CAD build for the part. Positions are in the model's coordinates, mm. A direction names the side the tool comes from. Give positions to 0.01 mm unless a question says otherwise; leave off trailing zeros. Write each loop counter-clockwise with the first axis right and the second up, starting at its lowest first coordinate (ties: lowest second). Pieces come first, ordered by that corner, then holes. Notation, with made-up numbers: (15.25, 48.5) - (24.25, 48.5) arc R12 ccw to (24.25, 68.5) - close; hole circle Ø5 at (61.5, 63.25). An arc over 180 degrees is marked (long way). Answer as a JSON object with one key per item and string values.
from build123d import *

# Parameters (mm, degrees)
SKETCH1_W            = 115
SKETCH1_H            = 100
BOSS_EXTRUDE1_DEPTH  = 20
SKETCH8_R            = 7
SKETCH8_R_2          = 6
BOSS_EXTRUDE4_DEPTH  = 20
SKETCH9_W            = 200
SKETCH9_H            = 100
BOSS_EXTRUDE5_DEPTH  = 16.6
SKETCH10_R           = 9
SKETCH10_R_2         = 10
BOSS_EXTRUDE7_DEPTH  = 20
SKETCH11_W           = 69.56
SKETCH11_H           = 59.638518518
SKETCH11_W_2         = 62.561838236
SKETCH11_H_2         = 53.638518518
BOSS_EXTRUDE9_DEPTH  = 15
SKETCH17_W           = 20
SKETCH17_H           = 100
BOSS_EXTRUDE15_DEPTH = 20
SKETCH15_R           = 14.1
CUT_EXTRUDE2_DEPTH   = 10
SKETCH21_R           = 1.76744544
SKETCH21_R_2         = 2.038433248
CUT_EXTRUDE3_DEPTH   = 20
SKETCH19_R           = 1.6
CUT_EXTRUDE4_DEPTH   = 38
CUT_EXTRUDE5_DEPTH   = 3
SKETCH23_W           = 7.97749669
SKETCH23_H           = 22.361861783
CUT_EXTRUDE6_DEPTH   = 10
CUT_EXTRUDE7_DEPTH   = 3
CUT_EXTRUDE8_DEPTH   = 3


with BuildPart() as part:
    # Sketch1 → Boss-Extrude1 (new body)
    with BuildSketch(Plane(origin=(0, 0, 0), x_dir=(1, 0, 0), z_dir=(0, 1, 0))):
        Rectangle(SKETCH1_W, SKETCH1_H)
    extrude(amount=BOSS_EXTRUDE1_DEPTH)

    # Sketch8 → Boss-Extrude4 (add)
    with BuildSketch(Plane.XZ):
        with Locations(Location((0, 0, 0), (0, 0, 90))):
            Circle(SKETCH8_R)
        with Locations(Location((42.407889557, -36.876425702, 0), (0, 0, 90))):
            Circle(SKETCH8_R_2)
        with Locations(Location((42.407889557, 36.876425702, 0), (0, 0, 90))):
            Circle(SKETCH8_R_2)
    extrude(amount=BOSS_EXTRUDE4_DEPTH)

    # Sketch9 → Boss-Extrude5 (add)
    with BuildSketch(Plane.XZ.offset(20)):
        with Locations((-42.5, 0)):
            Rectangle(SKETCH9_W, SKETCH9_H)
    extrude(amount=BOSS_EXTRUDE5_DEPTH)

    # Sketch10 → Boss-Extrude7 (add)
    with BuildSketch(Plane.XZ.offset(36.6)):
        with Locations(Location((37.5, -25, 0), (0, 0, 270))):
            Circle(SKETCH10_R)
        with Locations(Location((-122.5, -25, 0), (0, 0, 90))):
            Circle(SKETCH10_R)
        with Locations(Location((-122.5, 25, 0), (0, 0, 270))):
            Circle(SKETCH10_R)
        with Locations(Location((37.5, 25, 0), (0, 0, 90))):
            Circle(SKETCH10_R)
        with Locations(Location((-42.5, 0, 0), (0, 0, 270))):
            Circle(SKETCH10_R_2)
    extrude(amount=BOSS_EXTRUDE7_DEPTH)

    # Sketch11 → Boss-Extrude9 (add)
    with BuildSketch(Plane(origin=(0, 20, 0), x_dir=(1, 0, 0), z_dir=(0, 1, 0))):
        Rectangle(SKETCH11_W, SKETCH11_H)
        Rectangle(SKETCH11_W_2, SKETCH11_H_2, mode=Mode.SUBTRACT)
    extrude(amount=BOSS_EXTRUDE9_DEPTH)

    # Sketch17 → Boss-Extrude15 (add)
    with BuildSketch(Plane.XZ):
        with Locations((-47.5, 0)):
            Rectangle(SKETCH17_W, SKETCH17_H)
    extrude(amount=BOSS_EXTRUDE15_DEPTH)

    # Sketch15 → Cut-Extrude2 (cut)
    with BuildSketch(Plane(origin=(0, -20, 0), x_dir=(1, 0, 0), z_dir=(0, 1, 0))):
        with Locations(Location((-78.6, 0, 0), (0, 0, 270))):
            Circle(SKETCH15_R)
    extrude(amount=-CUT_EXTRUDE2_DEPTH, mode=Mode.SUBTRACT)

    # Sketch21 → Cut-Extrude3 (cut)
    with BuildSketch(Plane(origin=(0, -30, 0), x_dir=(1, 0, 0), z_dir=(0, 1, 0))):
        with Locations(Location((-85.16065049, 0, 0), (0, 0, 270))):
            Circle(SKETCH21_R)
        with Locations(Location((-73.222056531, 0, 0), (0, 0, 270))):
            Circle(SKETCH21_R_2)
    extrude(amount=-CUT_EXTRUDE3_DEPTH, mode=Mode.SUBTRACT)

    # Sketch19 → Cut-Extrude4 (cut)
    with BuildSketch(Plane.ZY.offset(57.5)):
        with Locations((-32.14, -13.409140004)):
            Circle(SKETCH19_R)
        with Locations((32.14, -13.409140004)):
            Circle(SKETCH19_R)
        with Locations((-32.14, 14.690859996)):
            Circle(SKETCH19_R)
        with Locations(Location((32.14, 14.690859996, 0), (0, 0, 180))):
            Circle(SKETCH19_R)
    extrude(amount=-CUT_EXTRUDE4_DEPTH, mode=Mode.SUBTRACT)

    # Sketch22 → Cut-Extrude5 (cut)
    with BuildSketch(Plane(origin=(-37.5, 0, 0), x_dir=(0, 0, -1), z_dir=(1, 0, 0))):
        Polygon((-29.09, -13.409140004), (-30.615, -10.767762522), (-33.665, -10.767762522), (-35.19, -13.409140004), (-33.665, -16.050517485), (-30.615, -16.050517485), align=None)
        Polygon((30.615, -16.050517485), (29.09, -13.409140004), (30.615, -10.767762522), (33.665, -10.767762522), (35.19, -13.409140004), (33.665, -16.050517485), align=None)
    extrude(amount=-CUT_EXTRUDE5_DEPTH, mode=Mode.SUBTRACT)

    # Sketch23 → Cut-Extrude6 (cut)
    with BuildSketch(Plane(origin=(0, 20, 0), x_dir=(1, 0, 0), z_dir=(0, 1, 0))):
        with Locations((-43.602813804, -38.819069109)):
            Rectangle(SKETCH23_W, SKETCH23_H)
        with Locations((-43.602813804, 38.819069109)):
            Rectangle(SKETCH23_W, SKETCH23_H)
    extrude(amount=-CUT_EXTRUDE6_DEPTH, mode=Mode.SUBTRACT)

    # Sketch24 → Cut-Extrude7 (cut)
    with BuildSketch(Plane(origin=(-47.591562149, 0, 0), x_dir=(0, 0, -1), z_dir=(1, 0, 0))):
        Polygon((-33.665, 17.332237478), (-35.19, 14.690859996), (-33.665, 12.049482515), (-30.615, 12.049482515), (-29.09, 14.690859996), (-30.615, 17.332237478), align=None)
    extrude(amount=-CUT_EXTRUDE7_DEPTH, mode=Mode.SUBTRACT)

    # Sketch25 → Cut-Extrude8 (cut)
    with BuildSketch(Plane(origin=(-47.591562149, 0, 0), x_dir=(0, 0, -1), z_dir=(1, 0, 0))):
        Polygon((35.19, 14.690859996), (33.665, 17.332237478), (30.615, 17.332237478), (29.09, 14.690859996), (30.615, 12.049482515), (33.665, 12.049482515), align=None)
    extrude(amount=-CUT_EXTRUDE8_DEPTH, mode=Mode.SUBTRACT)


solid = part.part
Item 1: Probe line 1 (X direction, y = -33.25, z = 0); line 2 (Y direction, x = -55, z = -32.14); line 3 (Y direction, x = -25.25, z = -32.14). List the from-to ranges inside material, lowest first. Write a range as from..to.
Entries:
{"line 1": "-142.5..-86.93, -83.39..-75.26, -71.18..57.5", "line 2": "-36.6..-15.01, -11.81..13.09, 16.29..20", "line 3": "-36.6..-20, 0..13.09, 16.29..20"}
Item 2: Cut at D-D (x = -128.5). Give the cut face in (y, z).
Entries:
{"outline": "(-56.6, -31.71) - (-36.6, -31.71) - (-36.6, -50) - (-20, -50) - (-20, 50) - (-36.6, 50) - (-36.6, 31.71) - (-56.6, 31.71) - (-56.6, 18.29) - (-36.6, 18.29) - (-36.6, -18.29) - (-56.6, -18.29) - close"}
Item 3: Mould opens along Z. For faces 1 (the flat face through (-21.7, -20.5, -50)), 2 (the cylindrical face through (-130.485, -46.46, 20.847)), 3 (the flat face through (-37.5, -10, -1)) say: +Z half, -Z half, draft (parallel to the pull), parting line (faces both ways), or undercut.
Entries:
{"face 1": "-Z half", "face 2": "undercut", "face 3": "draft"}
Item 4: Cut at B-B (x = -42.5). Give the cut face in (y, z), and give its area (3 significant figures).
Entries:
{"outline": "(-56.6, -10) - (-36.6, -10) - (-36.6, -50) - (10, -50) - (10, -27.64) - (20, -27.64) - (20, 27.64) - (10, 27.64) - (10, 50) - (-36.6, 50) - (-36.6, 10) - (-56.6, 10) - close; hole circle Ø3.2 at (-13.41, -32.14); hole circle Ø3.2 at (-13.41, 32.14)", "area": "5,600 mm2"}
Item 5: Which spindle directions (+Z, -Z, +X, -X, +Y, -Y) get a long thin tool onto all of the face, cutting with end or side? Do faces 4 (the flat face through (-44, 15, -27.638)), 5 (the flat face through (0, 20, 0)), 6 (the flat face through (-44, 15, 27.638)), 7 (the flat face through (-50.592, 15.9, 30.8)), 8 (the cylindrical face through (29.91, -46.46, 29.84)). Say none if no direction does.
Entries:
{"face 4": "-Z, +Y", "face 5": "+Y", "face 6": "+Z, +Y", "face 7": "none", "face 8": "-Y"}
Item 6: Cut at A-A (y = -43.5). Give the cut face in (x, z), and give its area (3 significant figures).
Entries:
{"outline": "circle Ø18 at (-122.5, -25); circle Ø18 at (-122.5, 25); circle Ø20 at (-42.5, 0); circle Ø18 at (37.5, -25); circle Ø18 at (37.5, 25)", "area": "1,330 mm2"}
Item 7: Cut at C-C (y = -24.5). Give the cut face in (x, z), and give its area (3 significant figures).
Entries:
{"outline": "(-142.5, -50) - (57.5, -50) - (57.5, 50) - (-142.5, 50) - close; hole circle Ø28.2 at (-78.6, 0)", "area": "19,400 mm2"}
Item 8: Flat gauge pins, fed straight in: P1, Ø1.6, axis at y = 15, z = 32.5, coming from the -X side; P2, Ø14, axis at x = -74, z = -5, coming from the +Y side; P3, Ø1, axis at x = 26.5, z = 11.5, coming from the +Y side; P4, Ø6.5, axis at x = -44.5, y = 16.5, coming from the +Z side. Where does each tip first touch, or does it go through?
Entries:
{"P1": "x = -19.5", "P2": "y = -30", "P3": "y = 20", "P4": "z = 50"}
